```python
from build123d import *

# Parameters (mm, degrees)
F0_W     = 160
F0_H     = 30
F1_DEPTH = 860
F2_R     = 2
F3_W     = 2
F3_H     = 30
F3_W_2   = 78
F4_DEPTH = 30.001


with BuildPart() as f1:
    # F0 (on Top) → F1 (new body, symmetric)
    with BuildSketch(Plane.XY):
        Rectangle(F0_W, F0_H)
    extrude(amount=F1_DEPTH, both=True)

    # F2
    f2_edges = [f1.edges().sort_by_distance(p)[0] for p in [
        (0, -15, -860),
        (80, -15, 0),
        (0, -15, 860),
        (-80, -15, 0),
        (80, 0, -860),
        (80, 15, 0),
        (80, 0, 860),
        (0, 15, 860),
        (-80, 0, 860),
        (0, 15, -860),
        (-80, 15, 0),
        (-80, 0, -860),
    ]]
    fillet(f2_edges, radius=F2_R)

    # F3 (on face) → F4 (cut, through all)
    with BuildSketch(Plane.XZ.offset(15)):
        with Locations((-79, -815)):
            Rectangle(F3_W, F3_H)
        with Locations((-39, -815)):
            Rectangle(F3_W_2, F3_H)
        with Locations((-79, 815)):
            Rectangle(F3_W, F3_H)
        with Locations((-39, 815)):
            Rectangle(F3_W_2, F3_H)
    extrude(amount=-F4_DEPTH, mode=Mode.SUBTRACT)


solid = f1.part
```
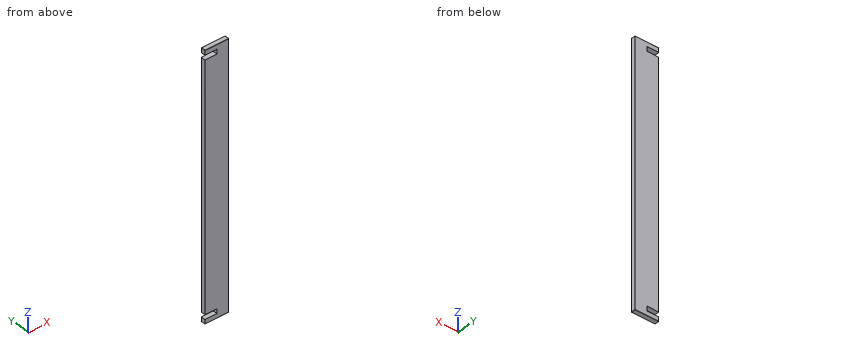
Source: CAD feature listing. Evaluate the final solid. Frame: model axes, mm. Coordinates: 2 decimals unless noted, no trailing zeros. Loops run counter-clockwise (first coordinate to the right, second up) from the corner with the lowest first, then second, coordinate; pieces in that order, holes last. Notation, with made-up numbers: (77, 28) - (108, 28) arc R26 cw to (108, 49) - close; hole circle Ø5 at (-16, 73). An arc over 180 degrees is marked (long way). Answer as CSV lines item,"result".
1. Section A-A (x = -33.5). Return loops of the section in (y, z), then the cut area to 3 significant figures.
Established:
outline,"(-15, -858) arc R2 ccw to (-13, -860) - (13, -860) arc R2 ccw to (15, -858) - (15, -830) - (-15, -830) - close; (-15, -800) - (15, -800) - (15, 800) - (-15, 800) - close; (-15, 830) - (15, 830) - (15, 858) arc R2 ccw to (13, 860) - (-13, 860) arc R2 ccw to (-15, 858) - close"
area,"49,800 mm2"
2. Ray query, line 1 (Z direction, x = -35.5, y = 1.25). Return the intervals inside material, ascending.
Established:
line 1,"z = -860 to -830, -800 to 800, 830 to 860"
3. Contact query for a flat-ended pin moving along its axis: pin 1 (9 mm diameter, centred on y = 2.5, z = -817.5, fed in from -X). Output: stop coordinate, or through.
Established:
pin 1,"stops at x = 0"
4. Section B-B (y = -1.25). Return loops of the section in (x, z), then the cut area to 3 significant figures.
Established:
outline,"(-80, -858) arc R2 ccw to (-78, -860) - (78, -860) arc R2 ccw to (80, -858) - (80, 858) arc R2 ccw to (78, 860) - (-78, 860) arc R2 ccw to (-80, 858) - (-80, 830) - (0, 830) - (0, 800) - (-80, 800) - (-80, -800) - (0, -800) - (0, -830) - (-80, -830) - close"
area,"270,000 mm2"
